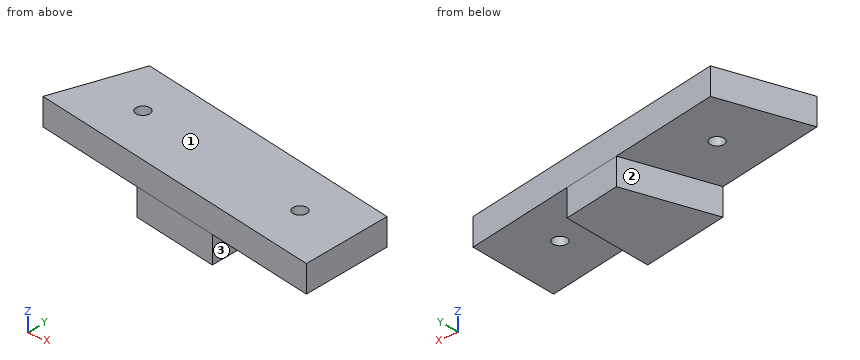
from build123d import *

# Parameters (mm, degrees)
EXTRUDE_1_DEPTH     = 6
EXTRUDE_2_DEPTH     = 6
SKETCH_3_R          = 1.55
CUT_EXTRUDE_1_DEPTH = 7


with BuildPart() as part:
    # Эскиз1 → Бобышка-Вытянуть1 (new body)
    with BuildSketch(Plane.XY):
        Polygon((-114.323496858, 125.813994573), (-183.895105895, 137.75282099), (-177.039061357, 157.140809371), (-114.323496858, 146.378513535), align=None)
    extrude(amount=EXTRUDE_1_DEPTH)

    # Эскиз2 → Бобышка-Вытянуть2 (add)
    with BuildSketch(Plane(origin=(0, 0, 0), x_dir=(-1, 0, 0), z_dir=(0, 0, -1))):
        Polygon((139.160448137, 150.64065515), (139.160448137, 130.076136187), (159.058154615, 133.490679376), (152.202110077, 152.878667757), align=None)
    extrude(amount=EXTRUDE_2_DEPTH)

    # Эскиз3 → Вырез-Вытянуть1 (cut, through all)
    with BuildSketch(Plane(origin=(0, 0, 0), x_dir=(-1, 0, 0), z_dir=(0, 0, -1))):
        with Locations((126.643413167, 138.210411601)):
            Circle(SKETCH_3_R)
        with Locations((168.147167316, 145.332657634)):
            Circle(SKETCH_3_R)
    extrude(amount=-CUT_EXTRUDE_1_DEPTH, mode=Mode.SUBTRACT)


solid = part.part
Could you check a few things on this model? Use its own coordinates, in mm. Face numbers are marked on the shaded views. A direction names the side the tool comes from. Coordinates: 2 decimals unless noted, no trailing zeros. Loops run counter-clockwise (first coordinate to the right, second up) from the corner with the lowest first, then second, coordinate; pieces in that order, holes last.
1. Imagine slicing it at B-B (y = 142). Please give me the cut outline in (x, z).
2. Imagine slicing it at D-D (z = 5). Please give me the cut outline in (x, y), and give its area (3 significant figures).
3. For P1, Ø5, axis at x = -134, z = -4.5, coming from the +Y side; P2, Ø7.5, axis at x = -131, y = 140.5, coming from the -Z side; P3, Ø1.8, axis at y = 145, z = -4.5, coming from the +X side; P4, Ø1.5, axis at x = -159, z = -4.5, coming from the -Y side, each with a flat end and sliding along its axis, tell me the tip position at first contact or that it passes through.
4. For the marked faces 1, 2 and 3, which set-ups out of +Z, -Z, +X, -X, +Y, -Y let a thin tool reach every point of the face, with its end or its side?
5. Imagine slicing it at C-C (x = -155). Please give me the cut outline in (y, z).
6. I need wall thicknesses on L1, parallel to Z at x = -121, y = 137; L2, parallel to Y at x = -132, z = 2.5; L3, parallel to Y at x = -136, z = 4.5. Which ranges of each line are inside material? Lowest first, please.
7. Imagine slicing it at A-A (z = -4). Please give me the cut outline in (x, y), and give its area (3 significant figures).
Computed values:
1. outline: (-182.39, 0) - (-156.05, 0) - (-156.05, -6) - (-139.16, -6) - (-139.16, 0) - (-114.32, 0) - (-114.32, 6) - (-182.39, 6) - close
2. outline: (-183.9, 137.75) - (-114.32, 125.81) - (-114.32, 146.38) - (-177.04, 157.14) - close; hole circle Ø3.1 at (-168.15, 145.33); hole circle Ø3.1 at (-126.64, 138.21)
2. area: 1,350 mm2
3. P1: passes through
3. P2: stops at z = 0
3. P3: stops at x = -139.16
3. P4: stops at y = 133.35
4. face 1: +Z, +X, -X, +Y, -Y
4. face 2: -Z, -X, +Y
4. face 3: -Z, +X, +Y, -Y
5. outline: (132.79, -6) - (144.97, -6) - (144.97, 0) - (153.36, 0) - (153.36, 6) - (132.79, 6) - close
6. L1: z = 0 to 6
6. L2: y = 128.85 to 149.41
6. L3: y = 129.53 to 150.1
7. outline: (-159.06, 133.49) - (-139.16, 130.08) - (-139.16, 150.64) - (-152.2, 152.88) - close
7. area: 339 mm2
